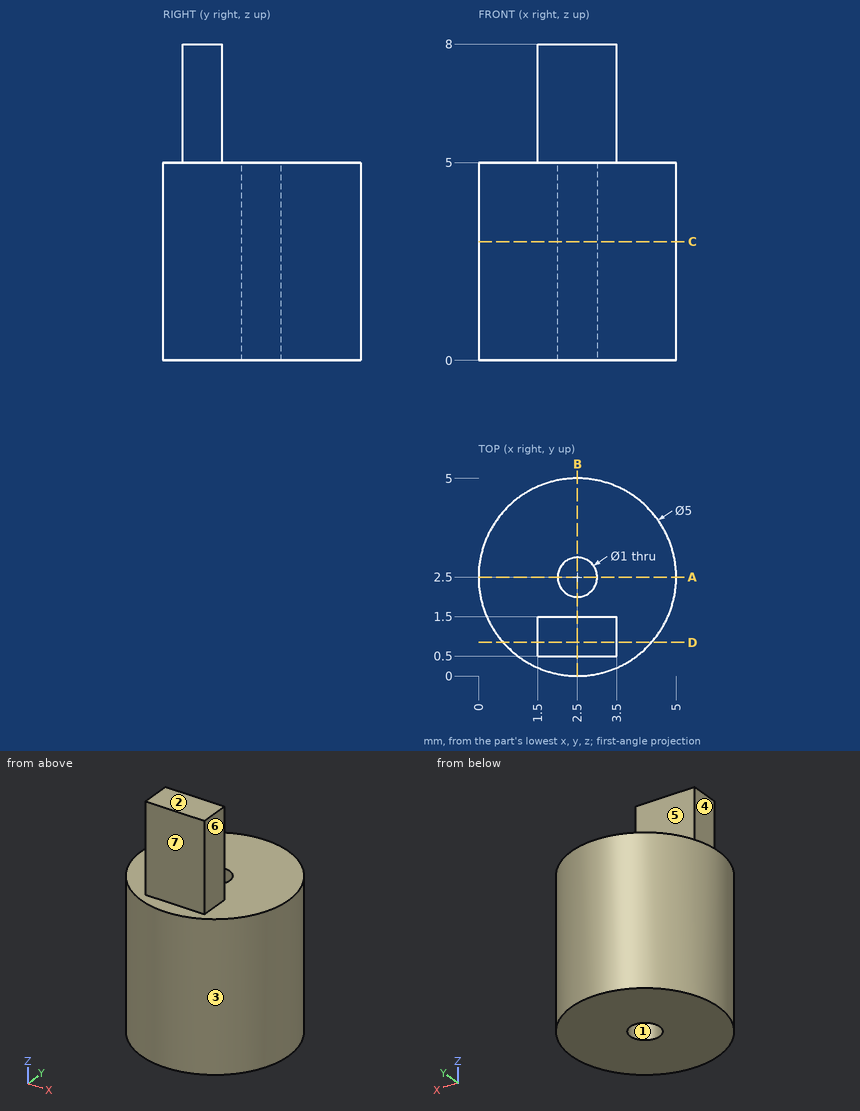
Study the drawing (mm; zero at the part's minimum x, y, z) and answer. A direction names the side the tool comes from. Coordinates: 2 decimals unless noted, no trailing zeros. Loops run counter-clockwise (first coordinate to the right, second up) from the corner with the lowest first, then second, coordinate; pieces in that order, holes last. Notation, with made-up numbers: M -12.5,-2.5 L 7.5,-2.5 A17 ccw 7.5,14.5 Z; hole C -35.5,-11 d9. An arc over 180 degrees is marked long. Answer in a Markdown table with one row per item. Add a question column.
1. Find section C-C, the plane z = 3. Write down the section's boundary in (x, y).
2. Find section A-A, the plane y = 2.5. Write down the section's boundary in (x, z), then the cut area to 3 significant figures.
3. Flat-ended cylindrical pins translate along their axes: P1, Ø1, axis at x = 2, z = 7, coming from the -Y side; P2, Ø0.5, axis at y = 1, z = 7, coming from the +X side; P3, Ø2, axis at x = 4, y = 3, coming from the +Z side. Find the tip coordinate at first contact, or state that the pin passes through.
4. Find section B-B, the plane x = 2.5. Write down the section's boundary in (y, z), then the cut area to 3 significant figures.
5. The mould has two halves that part along Y. Classify the marked faces 1, 2 and 3: pulls with the +Y half, pulls with the -Y half, needs draft (parallel to the pull), parting line crosses it, or undercut.
6. Find section D-D, the plane y = 0.85. Write down the section's boundary in (x, z), then the cut area to 3 significant figures.
7. A tool of negligible diameter and unlimited length cuts with its end or side. For the marked faces 4, 5, 6 and 7, from which of +Z, -Z, +X, -X, +Y, -Y can it reach the whole face along a straight path? Write none if from no direction.
8. Consider L1, parallel to X at y = 2.45, z = 1.75; L2, parallel to Y at x = 1.9, z = 6.25; L3, parallel to Z at x = 1.35, y = 2.6. Determine where each line is inside the solid, lowest interval first.
Reported:
| question | item | result |
|---|---|---|
| 1 | outline | C 2.5,2.5 d5; hole C 2.5,2.5 d1 |
| 2 | outline | M 0,0 L 2,0 L 2,5 L 0,5 Z; M 3,0 L 5,0 L 5,5 L 3,5 Z |
| 2 | area | 20.0 mm^2 |
| 3 | P1 | stops at y = 0.5 |
| 3 | P2 | stops at x = 3.5 |
| 3 | P3 | stops at z = 5 |
| 4 | outline | M 0,0 L 2,0 L 2,5 L 1.5,5 L 1.5,8 L 0.5,8 L 0.5,5 L 0,5 Z; M 3,0 L 5,0 L 5,5 L 3,5 Z |
| 4 | area | 23.0 mm^2 |
| 5 | face 1 | undercut |
| 5 | face 2 | needs draft |
| 5 | face 3 | parting line crosses it |
| 6 | outline | M 0.62,0 L 4.38,0 L 4.38,5 L 3.5,5 L 3.5,8 L 1.5,8 L 1.5,5 L 0.62,5 Z |
| 6 | area | 24.8 mm^2 |
| 7 | face 4 | +Z, -X, +Y, -Y |
| 7 | face 5 | +Z, +X, -X, +Y |
| 7 | face 6 | +Z, +X, +Y, -Y |
| 7 | face 7 | +Z, +X, -X, -Y |
| 8 | L1 | x = 0 to 2, 3 to 5 |
| 8 | L2 | y = 0.5 to 1.5 |
| 8 | L3 | z = 0 to 5 |
